CAD build for the part. Positions are in the model's coordinates, mm. A direction names the side the tool comes from. Coordinates: 2 decimals unless noted, no trailing zeros. Order: outer loops, then holes, each group sorted by start corner. A loop starts at its lowest first (then second) coordinate and runs counter-clockwise, first axis right, second up. Notation, with made-up numbers: M 0.25,61.5 L 45.25,61.5 A27 ccw 45.25,85.5 Z; hole C 21.5,25.25 d1. An arc over 180 degrees is marked long. One line per item, written item: value.
Autodesk Inventor part; units mm, degrees
ref_plane "YZ Plane" through (0, 0, 0) normal (1, 0, 0) x (0, 1, 0)
ref_plane "XZ Plane" through (0, 0, 0) normal (0, 1, 0) x (-1, 0, 0)
ref_plane "XY Plane" through (0, 0, 0) normal (0, 0, 1) x (1, 0, 0)
sketch "スケッチ1" plane through (0, 0, 0) normal (0, 1, 0) x (-1, 0, 0)
  line L0 (4, 0) -> (4, -3.5)
  line L1 (4, -3.5) -> (3, -3.5)
  line L2 (3, -3.5) -> (3, -2.5)
  line L3 (3, -2.5) -> (1, -2.5)
  line L4 (1, -2.5) -> (1, -3.5)
  line L5 (1, -3.5) -> (0, -3.5)
  line L6 (0, -3.5) -> (0, 0)
  line L7 (4, 0) -> (0, 0)
  line L8 (4, -1.5) -> (0, -1.5)
  dimension "d1" = 1
  dimension "d2" = 2
  dimension "d3" = 1.5
  dimension "d4" = 1
  dimension "d5" = 1
revolve "回転1" add sketch "スケッチ1" angle 360 about axis through (-4, 0, 0) along (1, 0, 0) contours L0 L1 L2 L3 L4 L5 L6 L8
properties part number "Pulley_MotorSide"
Q1. Slice it at D-D (z = -2). List the corners of the cut face in (x, y).
Recorded:
outline: M -4,-2.87 L -3,-2.87 L -3,-1.5 L -1,-1.5 L -1,-2.87 L 0,-2.87 L 0,2.87 L -1,2.87 L -1,1.5 L -3,1.5 L -3,2.87 L -4,2.87 Z
Q2. Slice it at A-A (z = 0). List the corners of the cut face in (x, y), plus the area to 3 significant figures.
Recorded:
outline: M -4,-3.5 L -3,-3.5 L -3,-2.5 L -1,-2.5 L -1,-3.5 L 0,-3.5 L 0,-1.5 L -4,-1.5 Z; M -4,1.5 L 0,1.5 L 0,3.5 L -1,3.5 L -1,2.5 L -3,2.5 L -3,3.5 L -4,3.5 Z
area: 12.0 mm^2
Q3. Pin check, flat tips, straight feed: pin 1 Ø1.5 at (x, z) = (-2, 0) entering from -Y; pin 2 Ø1.5 at (x, z) = (-3, 1) entering from +Y. Stop position of each tip, or through.
Recorded:
pin 1: stops at y = -2.5
pin 2: stops at y = 3.49
Q4. Which spindle directions (+Z, -Z, +X, -X, +Y, -Y) get a long thin tool onto all of the face, cutting with end or side? Do faces 1 (the face through (-4, -2, 0)), 2 (the face through (-3, -2, -2)). Say none if no direction does.
Recorded:
face 1: +Z, -Z, -X, +Y, -Y
face 2: none
Q5. Drill centre lines: line 1 along X through (y, z) = (0, -3); line 2 along Y through (x, z) = (-2.15, 0); line 3 along Y through (x, z) = (-3.1, 0). Where is each one in solid material? Low to high.
Recorded:
line 1: x = -4 to -3, -1 to 0
line 2: y = -2.5 to -1.5, 1.5 to 2.5
line 3: y = -3.5 to -1.5, 1.5 to 3.5
Q6. Mould opens along Z. For faces 3 (the face through (-1.97, 0.07, 1.5)), 4 (the face through (-3.493, -1.341, -3.233)), 5 (the face through (-1, -2, -2)) say: released by +Z, released by -Z, zero draft, split by the parting line, or undercut.
Recorded:
face 3: undercut
face 4: split by the parting line
face 5: zero draft
Q7. Slice it at C-C (x = -0.65). List the corners of the cut face in (y, z), plus the area to 3 significant figures.
Recorded:
outline: C 0,0 d7; hole C 0,0 d3
area: 31.4 mm^2
